Part print with two shaded views. Sizes in mm from the minimum x, y, z corner. Give positions to 0.01 mm unless a question says otherwise; leave off trailing zeros. Order: outer loops, then holes, each group sorted by start corner. A loop starts at its lowest first (then second) coordinate and runs counter-clockwise, first axis right, second up.
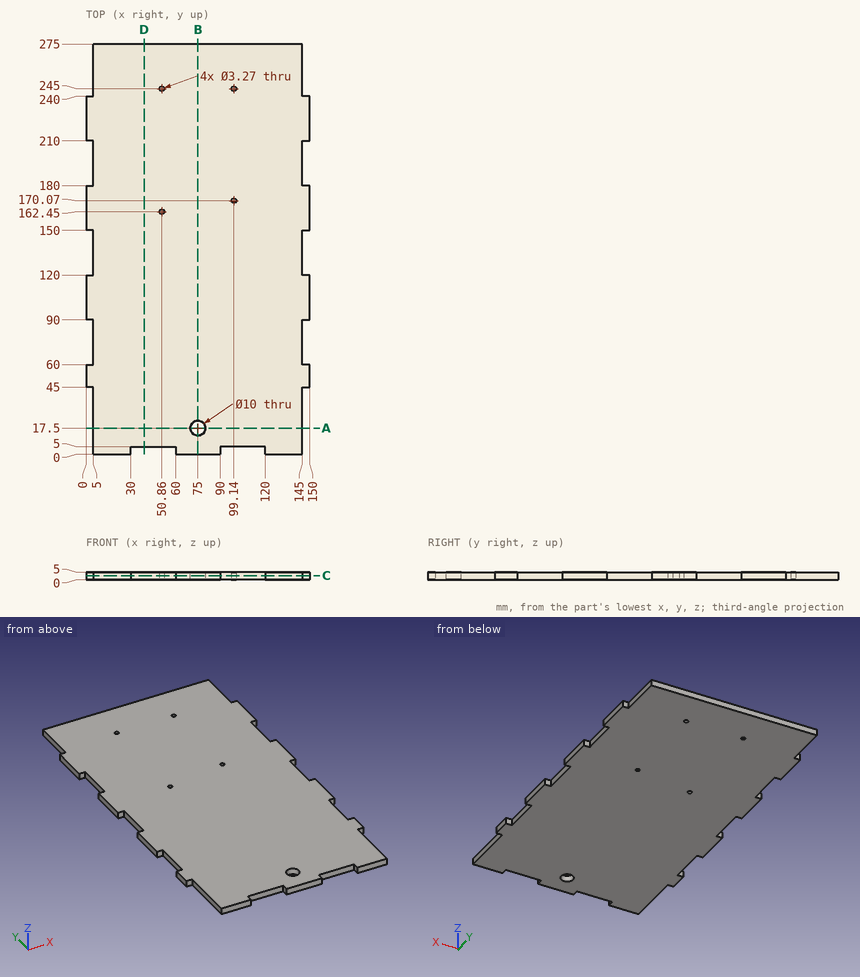
Item 1: Wall check: L1, parallel to X at y = 245, z = 4.05 (3 decimals); L2, parallel to Y at x = 99.14, z = 2.4 (3 decimals); L3, parallel to X at y = 170.07, z = 1.7 (3 decimals). Give the ranges that are in metal, low to high.
Item 2: Slice it at A-A (y = 17.5). Give the cut face in (x, z).
Item 3: Slice it at B-B (x = 75). Give the cut face in (y, z).
Item 4: Slice it at D-D (x = 39). Give the cut face in (y, z), and give its area (3 significant figures).
Item 5: Slice it at C-C (z = 2.7). State how many separate pieces and enclosed holes the cut face has, and give its area (3 significant figures).
Item 6: Drop flat-ended pins along their axis: pin 1 Ø2.5 at (x, y) = (50.86, 162.45) entering from +Z; pin 2 Ø1.5 at (y, z) = (21, 3.5) entering from +X; pin 3 Ø1.5 at (x, z) = (148, 1.5) entering from +Y; pin 4 Ø1 at (x, y) = (106.5, 203.5) entering from -Z. Give the stop position or say it passes through.
A:
1. L1: x = 5 to 49.225, 52.495 to 97.505, 100.775 to 145
1. L2: y = 5 to 168.435, 171.705 to 243.365, 246.635 to 275
1. L3: x = 0 to 97.505, 100.775 to 150
2. outline: (5, 0) - (70, 0) - (70, 5) - (5, 5) - close; (80, 0) - (145, 0) - (145, 5) - (80, 5) - close
3. outline: (0, 0) - (12.5, 0) - (12.5, 5) - (0, 5) - close; (22.5, 0) - (275, 0) - (275, 5) - (22.5, 5) - close
4. outline: (5, 0) - (275, 0) - (275, 5) - (5, 5) - close
4. area: 1,350 mm2
5. separate pieces: 1
5. enclosed holes: 5
5. area: 39,100 mm2
6. pin 1: passes through
6. pin 2: stops at x = 145
6. pin 3: stops at y = 240
6. pin 4: stops at z = 0
